The model under review builds one solid part; all positions refer to its coordinate system, in mm. A direction names the side the tool comes from. Give positions to 0.01 mm unless a question says otherwise; leave off trailing zeros. Loops run counter-clockwise (first coordinate to the right, second up) from the corner with the lowest first, then second, coordinate; pieces in that order, holes last. Notation, with made-up numbers: M 63,66.5 L 67,66.5 A8 cw 67,79.5 Z; hole C 46.5,35.25 d7. An arc over 180 degrees is marked long. Return JSON: item names as keys, results as strings.
```python
from build123d import *

# Parameters (mm, degrees)
F0_R     = 1.6
F0_R_2   = 1.575
F0_R_3   = 1.15
F0_R_4   = 5
F1_DEPTH = 5


with BuildPart() as f1:
    # F0 (on Top) → F1 (new body)
    with BuildSketch(Plane.XY):
        with BuildLine():
            Line((-93.5566243293, -2.4999999943), (-48.9433756768, -79.7724133547))
            ThreePointArc((-48.9433756768, -79.7724133547), (-47.1132486579, -81.6025403736), (-44.6132486579, -82.2724133548))
            Line((-44.6132486579, -82.2724133548), (44.6132486502, -82.2724133566))
            ThreePointArc((44.6132486502, -82.2724133566), (47.1132486502, -81.6025403755), (48.9433756692, -79.7724133566))
            Line((48.9433756692, -79.7724133566), (93.5566243248, -2.499999998))
            ThreePointArc((93.5566243248, -2.499999998), (94.2264973059, 2e-09), (93.5566243249, 2.500000002))
            Line((93.5566243249, 2.500000002), (48.9433756724, 79.7724133624))
            ThreePointArc((48.9433756724, 79.7724133624), (47.1132486535, 81.6025403814), (44.6132486535, 82.2724133625))
            Line((44.6132486535, 82.2724133625), (-44.6132486546, 82.2724133643))
            ThreePointArc((-44.6132486546, 82.2724133643), (-47.1132486546, 81.6025403832), (-48.9433756736, 79.7724133644))
            Line((-48.9433756736, 79.7724133644), (-93.5566243292, 2.5000000057))
            ThreePointArc((-93.5566243292, 2.5000000057), (-94.2264973103, 5.7e-09), (-93.5566243293, -2.4999999943))
        make_face()
        with Locations((-57.3397459654, -45.229473422)):
            Circle(F0_R, mode=Mode.SUBTRACT)
        with Locations((-43.4000000039, -75.1710050514)):
            Circle(F0_R_2, mode=Mode.SUBTRACT)
        with Locations((-27.0429399416, -67.839745966)):
            Circle(F0_R, mode=Mode.SUBTRACT)
        with Locations((-10.4999999994, -72.2724133636)):
            Circle(F0_R, mode=Mode.SUBTRACT)
        with Locations((-45.229473421, -57.339745966)):
            Circle(F0_R, mode=Mode.SUBTRACT)
        with Locations((-10.4999999994, -52.2724133636)):
            Circle(F0_R, mode=Mode.SUBTRACT)
        with Locations((-17.0429399416, -50.5192378903)):
            Circle(F0_R, mode=Mode.SUBTRACT)
        with Locations((-67.8397459654, -27.0429399426)):
            Circle(F0_R, mode=Mode.SUBTRACT)
        with Locations((-72.2724133636, -10.5000000006)):
            Circle(F0_R, mode=Mode.SUBTRACT)
        with Locations((-86.8000000044, 1.9e-09)):
            Circle(F0_R_2, mode=Mode.SUBTRACT)
        with Locations((-50.5192378897, -17.0429399426)):
            Circle(F0_R, mode=Mode.SUBTRACT)
        with Locations((-52.2724133636, -10.5000000006)):
            Circle(F0_R, mode=Mode.SUBTRACT)
        with Locations((-40.0192378897, -35.229473422)):
            Circle(F0_R, mode=Mode.SUBTRACT)
        with Locations((-35.229473421, -40.0192378903)):
            Circle(F0_R, mode=Mode.SUBTRACT)
        with Locations((-32.5, -32.5)):
            Circle(F0_R, mode=Mode.SUBTRACT)
        with Locations((-6.5, -27)):
            Circle(F0_R_3, mode=Mode.SUBTRACT)
        with Locations((-15.25, -15.25)):
            Circle(F0_R, mode=Mode.SUBTRACT)
        with Locations((10.5000000006, -72.2724133636)):
            Circle(F0_R, mode=Mode.SUBTRACT)
        with Locations((43.4000000006, -75.1710050533)):
            Circle(F0_R_2, mode=Mode.SUBTRACT)
        with Locations((27.0429399426, -67.8397459654)):
            Circle(F0_R, mode=Mode.SUBTRACT)
        with Locations((10.5000000006, -52.2724133636)):
            Circle(F0_R, mode=Mode.SUBTRACT)
        with Locations((17.0429399426, -50.5192378897)):
            Circle(F0_R, mode=Mode.SUBTRACT)
        with Locations((45.229473422, -57.3397459654)):
            Circle(F0_R, mode=Mode.SUBTRACT)
        with Locations((57.339745966, -45.229473421)):
            Circle(F0_R, mode=Mode.SUBTRACT)
        with Locations((6.5, -27)):
            Circle(F0_R_3, mode=Mode.SUBTRACT)
        with Locations((35.229473422, -40.0192378897)):
            Circle(F0_R, mode=Mode.SUBTRACT)
        with Locations((32.5, -32.5)):
            Circle(F0_R, mode=Mode.SUBTRACT)
        with Locations((40.0192378903, -35.229473421)):
            Circle(F0_R, mode=Mode.SUBTRACT)
        with Locations((15.25, -15.25)):
            Circle(F0_R, mode=Mode.SUBTRACT)
        Circle(F0_R_4, mode=Mode.SUBTRACT)
        with BuildLine():
            ThreePointArc((23.25, 6), (23.8357864376, 7.4142135624), (25.25, 8))
            Line((25.25, 8), (30.25, 8))
            ThreePointArc((30.25, 8), (31.6642135624, 7.4142135624), (32.25, 6))
            Line((32.25, 6), (32.25, -6))
            ThreePointArc((32.25, -6), (31.6642135624, -7.4142135624), (30.25, -8))
            Line((30.25, -8), (25.25, -8))
            ThreePointArc((25.25, -8), (23.8357864376, -7.4142135624), (23.25, -6))
            Line((23.25, -6), (23.25, 6))
        make_face(mode=Mode.SUBTRACT)
        with Locations((67.839745966, -27.0429399416)):
            Circle(F0_R, mode=Mode.SUBTRACT)
        with Locations((50.5192378903, -17.0429399416)):
            Circle(F0_R, mode=Mode.SUBTRACT)
        with Locations((52.2724133636, -10.4999999994)):
            Circle(F0_R, mode=Mode.SUBTRACT)
        with Locations((72.2724133636, -10.4999999994)):
            Circle(F0_R, mode=Mode.SUBTRACT)
        with Locations((86.8000000044, -1.9e-09)):
            Circle(F0_R_2, mode=Mode.SUBTRACT)
        with Locations((-72.2724133636, 10.4999999994)):
            Circle(F0_R, mode=Mode.SUBTRACT)
        with Locations((-52.2724133636, 10.4999999994)):
            Circle(F0_R, mode=Mode.SUBTRACT)
        with Locations((-50.5192378903, 17.0429399416)):
            Circle(F0_R, mode=Mode.SUBTRACT)
        with Locations((-67.839745966, 27.0429399416)):
            Circle(F0_R, mode=Mode.SUBTRACT)
        with Locations((-15.25, 15.25)):
            Circle(F0_R, mode=Mode.SUBTRACT)
        with Locations((-40.0192378903, 35.229473421)):
            Circle(F0_R, mode=Mode.SUBTRACT)
        with Locations((-32.5, 32.5)):
            Circle(F0_R, mode=Mode.SUBTRACT)
        with Locations((-35.229473422, 40.0192378897)):
            Circle(F0_R, mode=Mode.SUBTRACT)
        with Locations((-6.5, 27)):
            Circle(F0_R_3, mode=Mode.SUBTRACT)
        with Locations((-57.339745966, 45.229473421)):
            Circle(F0_R, mode=Mode.SUBTRACT)
        with Locations((-45.229473422, 57.3397459654)):
            Circle(F0_R, mode=Mode.SUBTRACT)
        with Locations((-17.0429399426, 50.5192378897)):
            Circle(F0_R, mode=Mode.SUBTRACT)
        with Locations((-10.5000000006, 52.2724133636)):
            Circle(F0_R, mode=Mode.SUBTRACT)
        with Locations((-27.0429399426, 67.8397459654)):
            Circle(F0_R, mode=Mode.SUBTRACT)
        with Locations((-43.4000000006, 75.1710050533)):
            Circle(F0_R_2, mode=Mode.SUBTRACT)
        with Locations((-10.5000000006, 72.2724133636)):
            Circle(F0_R, mode=Mode.SUBTRACT)
        with Locations((15.25, 15.25)):
            Circle(F0_R, mode=Mode.SUBTRACT)
        with Locations((6.5, 27)):
            Circle(F0_R_3, mode=Mode.SUBTRACT)
        with Locations((32.5, 32.5)):
            Circle(F0_R, mode=Mode.SUBTRACT)
        with Locations((35.229473421, 40.0192378903)):
            Circle(F0_R, mode=Mode.SUBTRACT)
        with Locations((40.0192378897, 35.229473422)):
            Circle(F0_R, mode=Mode.SUBTRACT)
        with Locations((52.2724133636, 10.5000000006)):
            Circle(F0_R, mode=Mode.SUBTRACT)
        with Locations((50.5192378897, 17.0429399426)):
            Circle(F0_R, mode=Mode.SUBTRACT)
        with Locations((72.2724133636, 10.5000000006)):
            Circle(F0_R, mode=Mode.SUBTRACT)
        with Locations((67.8397459654, 27.0429399426)):
            Circle(F0_R, mode=Mode.SUBTRACT)
        with Locations((17.0429399416, 50.5192378903)):
            Circle(F0_R, mode=Mode.SUBTRACT)
        with Locations((10.4999999994, 52.2724133636)):
            Circle(F0_R, mode=Mode.SUBTRACT)
        with Locations((45.229473421, 57.339745966)):
            Circle(F0_R, mode=Mode.SUBTRACT)
        with Locations((10.4999999994, 72.2724133636)):
            Circle(F0_R, mode=Mode.SUBTRACT)
        with Locations((27.0429399416, 67.839745966)):
            Circle(F0_R, mode=Mode.SUBTRACT)
        with Locations((43.4000000039, 75.1710050514)):
            Circle(F0_R_2, mode=Mode.SUBTRACT)
        with Locations((57.3397459654, 45.229473422)):
            Circle(F0_R, mode=Mode.SUBTRACT)
        with Locations((-6.5, -27)):
            Circle(F0_R_3)
        with Locations((6.5, -27)):
            Circle(F0_R_3)
        with Locations((6.5, 27)):
            Circle(F0_R_3)
        with Locations((-6.5, 27)):
            Circle(F0_R_3)
        Circle(F0_R_4)
    extrude(amount=F1_DEPTH)


solid = f1.part
```
1) Wall thickness on L1, parallel to Y at x = 32.5, z = 3.8; L2, parallel to Y at x = -43.4, z = 3.4; L3, parallel to Y at x = -10.5, z = 2.6: over which ranges is each line inside the solid? List them lowest first. Write a range as from..to.
From the geometry:
{"L1": "-82.27..-34.1, -30.9..30.9, 34.1..82.27", "L2": "-82.27..-76.75, -73.6..73.6, 76.75..82.27", "L3": "-82.27..-73.87, -70.67..-53.87, -50.67..50.67, 53.87..70.67, 73.87..82.27"}
2) Consider section A-A on x = 80.5. Write out the cut boundary in (y, z).
From the geometry:
{"outline": "M -25.11,0 L 25.11,0 L 25.11,5 L -25.11,5 Z"}
3) Consider section B-B on z = 1.4. Count the separate pieces of the cut face and the enclosed holes in it, then the cut area to 3 significant figures.
From the geometry:
{"separate pieces": "1", "enclosed holes": "63", "area": "22,800 mm²"}
4) The part is to be moulded in two halves that separate along Y. For faces 3 (the face through (47.08, -81.62, 2.46)), 4 (the face through (-1, 1, 0)), 5 (the face through (23.25, 0, 2)), say which applies: released by +Y, released by -Y, zero draft, split by the parting line, or undercut.
From the geometry:
{"face 3": "released by -Y", "face 4": "zero draft", "face 5": "undercut"}
5) Tool access review of faces 1 (the face through (28, 8, 2)), 2 (the face through (-47.08, 81.62, 2.46)): name each direction out of +Z, -Z, +X, -X, +Y, -Y from which nothing blocks a thin tool from reaching the whole face with its end or side.
From the geometry:
{"face 1": "+Z, -Z", "face 2": "+Z, -Z, -X, +Y"}
6) Insertion check: pin 1 (2.5 mm diameter, centred on y = 2, z = 3.5, fed in from -X); pin 2 (6 mm diameter, centred on x = 25, y = 22.5, fed in from -Z); pin 3 (1.9 mm diameter, centred on x = -50.52, y = -17.04, fed in from +Z). Each pin has a flat end and moves straight along its axis. Give the tip position at first contact, or say it passes through.
From the geometry:
{"pin 1": "x = -94.17", "pin 2": "z = 0", "pin 3": "through"}
